Geometry: see drawing. Coordinates: mm, zero at the bounding-box minimum. A direction names the side the tool comes from. Coordinates: 2 decimals unless noted, no trailing zeros. Write each loop counter-clockwise with the first axis right and the second up, starting at its lowest first coordinate (ties: lowest second). Pieces come first, ordered by that corner, then holes. Notation, with made-up numbers: (-8.5, -17.75) - (37.5, -17.75) arc R21 ccw to (37.5, 16.25) - close; hole circle Ø10 at (-24, 82.25). An arc over 180 degrees is marked (long way). Use CSV: the item, a comma, the result in double quotes.
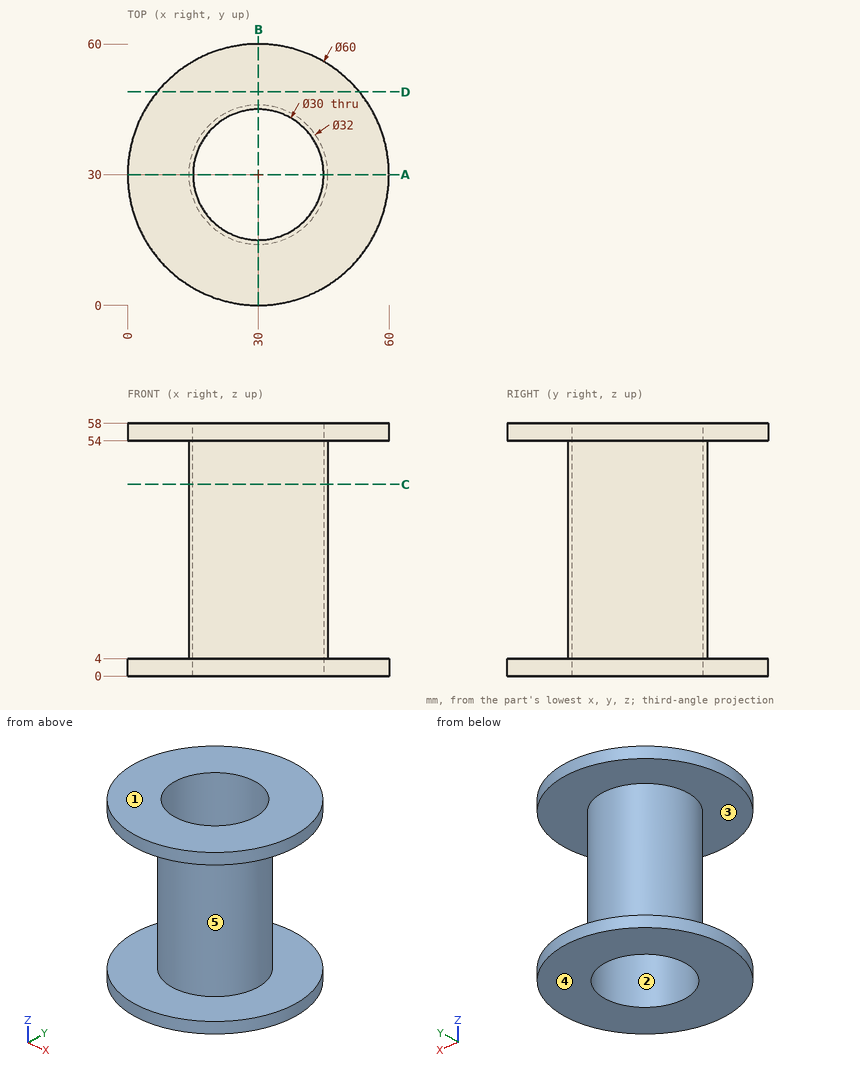
(1) Cut plane A-A on y = 30. Return loops of the section in (x, z), and give its area (3 significant figures).
Check values:
outline,"(0, 0) - (15, 0) - (15, 58) - (0, 58) - (0, 54) - (14, 54) - (14, 4) - (0, 4) - close; (45, 0) - (60, 0) - (60, 4) - (46, 4) - (46, 54) - (60, 54) - (60, 58) - (45, 58) - close"
area,"340 mm^2"
(2) Reachability of the marked faces 4 and 5 from +Z, -Z, +X, -X, +Y, -Y: full face, straight path, thin tool, end or side. Return the list, or none.
Check values:
face 4,"-Z, +X, -X, +Y, -Y"
face 5,"none"
(3) Draft query along Z for the marked faces 1, 2 and 3. Return one class per face: pulls with the +Z half, pulls with the -Z half, needs draft (parallel to the pull), parting line crosses it, or undercut.
Check values:
face 1,"pulls with the +Z half"
face 2,"needs draft"
face 3,"undercut"
(4) Ray query, probe 1 along Z at (x, y) = (50.5, 21); probe 2 along Y at (x, z) = (30, 39.5); probe 3 along Y at (x, z) = (21, 7.5). Return the intervals inside material, ascending. Write a range as from..to.
Check values:
probe 1,"0..4, 54..58"
probe 2,"14..15, 45..46"
probe 3,"16.77..18, 42..43.23"
(5) Pin query (flat end, axial travel): pin 1 Ø12 at (y, z) = (28, 23) entering from -X; pin 2 Ø1.5 at (x, z) = (38, 33) entering from -Y; pin 3 Ø2 at (y, z) = (45, 28.5) entering from +X; pin 4 Ø8 at (x, y) = (7, 53) entering from -Z. Return the tip coordinate at first contact, or that it passes through.
Check values:
pin 1,"x = 14"
pin 2,"y = 15.74"
pin 3,"x = 37.75"
pin 4,"z = 0"
(6) Cut plane C-C on z = 44. Return loops of the section in (x, y), and give its area (3 significant figures).
Check values:
outline,"circle Ø32 at (30, 30); hole circle Ø30 at (30, 30)"
area,"97.4 mm^2"
(7) Cut plane D-D on y = 49. Return loops of the section in (x, z), and give its area (3 significant figures).
Check values:
outline,"(6.78, 0) - (53.22, 0) - (53.22, 4) - (6.78, 4) - close; (6.78, 54) - (53.22, 54) - (53.22, 58) - (6.78, 58) - close"
area,"371 mm^2"
